Source: CAD feature listing. Evaluate the final solid. Frame: model axes, mm. A direction names the side the tool comes from. Coordinates: 2 decimals unless noted, no trailing zeros. Loops run counter-clockwise (first coordinate to the right, second up) from the corner with the lowest first, then second, coordinate; pieces in that order, holes last. Notation, with made-up numbers: (74.5, 60.5) -> (114.5, 60.5) arc R21 ccw to (114.5, 92.5) -> close; hole circle Ø10 at (57.25, 59.5). An arc over 180 degrees is marked (long way). Answer as a JSON object with one key per item and string values. Group by question number.
from build123d import *

# Parameters (mm, degrees)
F0_R     = 19.05
F1_DEPTH = 174.57928
F4_DEPTH = 20.828
F5_R     = 9.525
F6_DEPTH = 20.828
F7_SIZE2 = 1.524
F7_SIZE  = 1.524


with BuildPart() as f1:
    # F0 (on Front) → F1 (new body)
    with BuildSketch(Plane.XZ):
        Circle(F0_R)
    extrude(amount=F1_DEPTH)

    # F2 (on face) → F3 (revolve)
    with BuildSketch(Plane(origin=(0, 0, 0), x_dir=(-1, 0, 0), z_dir=(0, 1, 0))):
        with BuildLine():
            Line((19.05, 0), (0, 0))
            Line((0, 0), (0, -19.05))
            ThreePointArc((0, -19.05), (13.4703841816, -13.4703841816), (19.05, 0))
        make_face()
    revolve(axis=Axis((0, 0, -2.0931214094), (0, 0, -1)))

    # F4 (cut): a face of the model
    f4_faces = [f1.faces().sort_by_distance(p)[0] for p in [
        (0, 0, 8.0850711091),
    ]]
    extrude(f4_faces, amount=-F4_DEPTH, mode=Mode.SUBTRACT)

    # F5 (on face) → F6 (join)
    with BuildSketch(Plane.XY):
        Circle(F5_R)
    extrude(amount=F6_DEPTH)

    # F7
    f7_edges = [f1.edges().sort_by_distance(p)[0] for p in [
        (-9.525, 0, 20.828),
    ]]
    chamfer(f7_edges, length=F7_SIZE, length2=F7_SIZE2)


solid = f1.part
1. Pin query (flat end, axial travel): pin 1 Ø10 at (y, z) = (-146.5, -14) entering from -X; pin 2 Ø10 at (y, z) = (-105, -12) entering from -X; pin 3 Ø9.5 at (x, z) = (-1.5, 11.5) entering from +Y (3 decimals). Return the tip coordinate at first contact, or that it passes through.
2. Section query D-D on x = -15. Return loops of the section in (y, z).
3. Section query B-B on z = 2.5. Return loops of the section in (x, y) (3 decimals), then the cut area to 3 significant figures.
4. Mould query, pull axis Y, two halves, no side actions, for faces 1 (the face through (0, -174.579, 0)), 2 (the face through (-4.13, -86.068, -18.597)), 3 (the face through (-7.559, -5.796, 9.517)). Classes: pulls with the +Y half, pulls with the -Y half, needs draft (parallel to the pull), parting line crosses it, or undercut.
5. Ray query, L1, parallel to Y at x = -17, z = 2; L2, parallel to X at y = -30, z = 1. Return the intervals inside material, ascending.
6. Reachability of faces 4 (the face through (0, 0, 20.828)), 5 (the face through (0, -20.828, 8)), 6 (the face through (-4, -9, 0)) from +Z, -Z, +X, -X, +Y, -Y: full face, straight path, thin tool, end or side. Return the list, or none.
7. Section query A-A on x = 0. Return loops of the section in (y, z) (3 decimals).
8. Section query C-C on y = -135.5. Return loops of the section in (x, z), then the cut area to 3 significant figures.
Solved:
{
 "1": {"pin 1": "x = -16.79", "pin 2": "x = -17.72", "pin 3": "y = 9.525"},
 "2": {"outline": "(-174.58, -11.74) -> (0, -11.74) arc R11.74 ccw to (11.74, 0) -> (-20.83, 0) -> (-20.83, 11.74) -> (-174.58, 11.74) -> close"},
 "3": {"outline": "(-18.885, -174.579) -> (18.885, -174.579) -> (18.885, -20.828) -> (-18.885, -20.828) -> close; circle Ø19.05 at (0, 0)", "area": "6,090 mm^2"},
 "4": {"face 1": "pulls with the -Y half", "face 2": "needs draft", "face 3": "undercut"},
 "5": {"L1": "-174.58 to -20.83", "L2": "-19.02 to 19.02"},
 "6": {"face 4": "+Z, +X, -X, +Y, -Y", "face 5": "+Z, +X, -X", "face 6": "+Z"},
 "7": {"outline": "(-174.579, -19.05) -> (0, -19.05) arc R19.05 ccw to (19.05, 0) -> (9.525, 0) -> (9.525, 19.304) -> (8.001, 20.828) -> (-8.001, 20.828) -> (-9.525, 19.304) -> (-9.525, 0) -> (-20.828, 0) -> (-20.828, 19.05) -> (-174.579, 19.05) -> close"},
 "8": {"outline": "circle Ø38.1 at (0, 0)", "area": "1,140 mm^2"}
}
